from build123d import *

# Parameters (mm, degrees)
SKETCH1_R           = 2.6
BOSS_EXTRUDE1_DEPTH = 5
SKETCH2_W           = 69.749863317
SKETCH2_H           = 53.464567198
SKETCH2_W_2         = 56
SKETCH2_H_2         = 33
SKETCH2_R           = 13.5
CUT_EXTRUDE1_DEPTH  = 10
BOSS_EXTRUDE2_DEPTH = 5


with BuildPart() as part:
    # Sketch1 → Boss-Extrude1 (new body)
    with BuildSketch(Plane.XY):
        with BuildLine():
            Line((-28, -18.201493875), (-28, -24.201493875))
            Line((-28, -24.201493875), (28, -24.201493875))
            Line((28, -24.201493875), (28, -18.201493875))
            Line((28, -18.201493875), (26, -18.201493875))
            Line((26, -18.201493875), (26, -15.701493875))
            Line((26, -15.701493875), (23, -15.701493875))
            Line((23, -15.701493875), (23, -16.951493875))
            ThreePointArc((23, -16.951493875), (22, -17.951493875), (21, -16.951493875))
            Line((21, -16.951493875), (21, -15.701493875))
            Line((21, -15.701493875), (16, -15.701493875))
            Line((16, -15.701493875), (16, -12.701493875))
            Line((16, -12.701493875), (21, -12.701493875))
            Line((21, -12.701493875), (21, -11.451493875))
            ThreePointArc((21, -11.451493875), (22, -10.451493875), (23, -11.451493875))
            Line((23, -11.451493875), (23, -12.701493875))
            Line((23, -12.701493875), (26, -12.701493875))
            Line((26, -12.701493875), (26, -10.201493875))
            Line((26, -10.201493875), (28, -10.201493875))
            Line((28, -10.201493875), (28, -4.201493875))
            Line((28, -4.201493875), (26, -4.201493875))
            Line((26, -4.201493875), (26, 2.924352213))
            Line((26, 2.924352213), (12, 17.426918513))
            Line((12, 17.426918513), (-12, 17.426918513))
            Line((-12, 17.426918513), (-26, 2.924352213))
            Line((-26, 2.924352213), (-26, -4.201493875))
            Line((-26, -4.201493875), (-28, -4.201493875))
            Line((-28, -4.201493875), (-28, -10.201493875))
            Line((-28, -10.201493875), (-26, -10.201493875))
            Line((-26, -10.201493875), (-26, -12.701493875))
            Line((-26, -12.701493875), (-23, -12.701493875))
            Line((-23, -12.701493875), (-23, -11.451493875))
            ThreePointArc((-23, -11.451493875), (-22, -10.451493875), (-21, -11.451493875))
            Line((-21, -11.451493875), (-21, -12.701493875))
            Line((-21, -12.701493875), (-16, -12.701493875))
            Line((-16, -12.701493875), (-16, -15.701493875))
            Line((-16, -15.701493875), (-21, -15.701493875))
            Line((-21, -15.701493875), (-21, -16.951493875))
            ThreePointArc((-21, -16.951493875), (-22, -17.951493875), (-23, -16.951493875))
            Line((-23, -16.951493875), (-23, -15.701493875))
            Line((-23, -15.701493875), (-26, -15.701493875))
            Line((-26, -15.701493875), (-26, -18.201493875))
            Line((-26, -18.201493875), (-28, -18.201493875))
        make_face()
        with Locations((-21.5, -6.201493875)):
            Circle(SKETCH1_R, mode=Mode.SUBTRACT)
        with Locations((21.5, -6.201493875)):
            Circle(SKETCH1_R, mode=Mode.SUBTRACT)
        with BuildLine():
            Line((8.25, 3.201632482), (8.25, -1.451493875))
            Line((8.25, -1.451493875), (3.596873642, -1.451493875))
            ThreePointArc((3.596873642, -1.451493875), (0, -2.201493875), (-3.596873642, -1.451493875))
            Line((-3.596873642, -1.451493875), (-8.25, -1.451493875))
            Line((-8.25, -1.451493875), (-8.25, 3.201632482))
            ThreePointArc((-8.25, 3.201632482), (-8.626766656, 4.233570052), (-8.875, 5.303723532))
            ThreePointArc((-8.875, 5.303723532), (-10.25, 6.798506125), (-8.875, 8.293288717))
            ThreePointArc((-8.875, 8.293288717), (-8.626766656, 9.363442197), (-8.25, 10.395379767))
            Line((-8.25, 10.395379767), (-8.25, 15.048506125))
            Line((-8.25, 15.048506125), (-3.596873642, 15.048506125))
            ThreePointArc((-3.596873642, 15.048506125), (0, 15.798506125), (3.596873642, 15.048506125))
            Line((3.596873642, 15.048506125), (8.25, 15.048506125))
            Line((8.25, 15.048506125), (8.25, 10.395379767))
            ThreePointArc((8.25, 10.395379767), (8.626766656, 9.363442197), (8.875, 8.293288717))
            ThreePointArc((8.875, 8.293288717), (10.25, 6.798506125), (8.875, 5.303723532))
            ThreePointArc((8.875, 5.303723532), (8.626766656, 4.233570052), (8.25, 3.201632482))
        make_face(mode=Mode.SUBTRACT)
    extrude(amount=BOSS_EXTRUDE1_DEPTH)

    # Sketch2 → Cut-Extrude1 (cut)
    # profile 1 of 2: a face of its own
    with BuildSketch(Plane.XY.offset(5)):
        with Locations((5.197554668, -6.913421349)):
            Rectangle(SKETCH2_W, SKETCH2_H)
        with Locations((0, -14.201493875)):
            Rectangle(SKETCH2_W_2, SKETCH2_H_2, mode=Mode.SUBTRACT)
    # profile 2 of 2: a face of its own
    with BuildSketch(Plane.XY.offset(5)):
        with Locations((0, -14.201493875)):
            Circle(SKETCH2_R)
    extrude(amount=-CUT_EXTRUDE1_DEPTH, mode=Mode.SUBTRACT)


with BuildPart() as cut_extrude1_piece_1:
    # of the separate pieces the step leaves, piece 1, a body of its own (cut_extrude1_pieces)
    add(part.part.solids().sort_by_distance((9.069178574, -24.201493875, 0))[0])



with BuildPart() as cut_extrude1_piece_2:
    # of the separate pieces the step leaves, piece 2, a body of its own (cut_extrude1_pieces)
    add(part.part.solids().sort_by_distance((-28, -18.201493875, 0))[0])


with BuildPart() as cut_extrude1_piece_1_1:
    add(cut_extrude1_piece_1.part)

    add(cut_extrude1_piece_2.part)  # Boss-Extrude2 merges Cut-Extrude1 piece 2
    # Sketch3 → Boss-Extrude2 (add)
    with BuildSketch(Plane(origin=(0, 0, 0), x_dir=(-1, 0, 0), z_dir=(0, 0, -1))):
        with BuildLine():
            Line((-26, -4.201493875), (-26, -0.701493875))
            Line((-26, -0.701493875), (-26, 2.298506125))
            Line((-26, 2.298506125), (-8.25, 2.298506125))
            Line((-8.25, 2.298506125), (-8.25, -0.701493875))
            Line((-8.25, -0.701493875), (-8.25, -1.451493875))
            Line((-8.25, -1.451493875), (-4.437059837, -1.451493875))
            ThreePointArc((-4.437059837, -1.451493875), (2.167902598, -0.876697505), (8.25, -3.515638739))
            Line((8.25, -3.515638739), (8.25, -0.701493875))
            Line((8.25, -0.701493875), (26, -0.701493875))
            Line((26, -0.701493875), (26, -4.201493875))
            Line((26, -4.201493875), (28, -4.201493875))
            Line((28, -4.201493875), (28, -0.701493875))
            Line((28, -0.701493875), (28, 4.298506125))
            Line((28, 4.298506125), (-28.241259843, 4.298506125))
            Line((-28.241259843, 4.298506125), (-28.241259843, -0.701493875))
            Line((-28.241259843, -0.701493875), (-28.241259843, -4.201493875))
            Line((-28.241259843, -4.201493875), (-28, -4.201493875))
            Line((-28, -4.201493875), (-26, -4.201493875))
        make_face()
        Polygon((28, -27.701493875), (0, -27.701493875), (-28, -27.701493875), (-28, -32.701493875), (28, -32.701493875), align=None)
        with BuildLine():
            Line((28, -24.201493875), (9.069178574, -24.201493875))
            ThreePointArc((9.069178574, -24.201493875), (4.860555524, -26.796135593), (0, -27.701493875))
            Line((0, -27.701493875), (28, -27.701493875))
            Line((28, -27.701493875), (28, -24.201493875))
        make_face()
        with BuildLine():
            ThreePointArc((0, -27.701493875), (-4.860555524, -26.796135593), (-9.069178574, -24.201493875))
            Line((-9.069178574, -24.201493875), (-28, -24.201493875))
            Line((-28, -24.201493875), (-28, -27.701493875))
            Line((-28, -27.701493875), (0, -27.701493875))
        make_face()
    extrude(amount=-BOSS_EXTRUDE2_DEPTH)


solid = cut_extrude1_piece_1_1.part
Could you check a few things on this model? Use its own coordinates, in mm. A direction names the side the tool comes from. Coordinates: 2 decimals unless noted, no trailing zeros. Order: outer loops, then holes, each group sorted by start corner. A loop starts at its lowest first (then second) coordinate and runs counter-clockwise, first axis right, second up. Notation, with made-up numbers: (-28.5, 16.5) -> (4.5, 16.5) arc R37 ccw to (4.5, 54.5) -> close; hole circle Ø4 at (26, 75). An arc over 180 degrees is marked (long way). One line per question, with ' | ' between items.
Q1. Thinking about a two-plate mould opening in X: for faces 1 (the face through (21, -16, 2)), 2 (the face through (13, -10, 5)), 3 (the face through (16, -14, 2)), which applies, pulls with the +X half, pulls with the -X half, needs draft (parallel to the pull), parting line crosses it, or undercut?
Return value:
face 1: undercut | face 2: needs draft | face 3: pulls with the +X half
Q2. Imagine slicing it at C-C on y = -26. Please give me the cut outline in (x, z), and give its area (3 significant figures).
Return value:
outline: (-28, 0) -> (-6.56, 0) -> (-6.56, 5) -> (-28, 5) -> close; (6.56, 0) -> (28, 0) -> (28, 5) -> (6.56, 5) -> close | area: 214 mm²
Q3. Imagine slicing it at A-A on x = -11. Please give me the cut outline in (y, z), and give its area (3 significant figures).
Return value:
outline: (-32.7, 0) -> (-22.03, 0) -> (-22.03, 5) -> (-32.7, 5) -> close; (-6.38, 0) -> (4.3, 0) -> (4.3, 5) -> (-6.38, 5) -> close | area: 107 mm²
Q4. Imagine slicing it at D-D on z = 1.2. State how many separate pieces and enclosed holes the cut face has, and give its area (3 significant figures).
Return value:
separate pieces: 1 | enclosed holes: 3 | area: 1,350 mm²
Q5. I'm going to push flat-ended pins straight in: P1, Ø3, axis at y = -16.5, z = 1.5, coming from the +X side; P2, Ø1.5, axis at y = -14.5, z = 1.5, coming from the -X side; P3, Ø7, axis at x = 21.5, y = -6.2, coming from the -Z side; P4, Ø0.6, axis at y = -12.5, z = 1.5, coming from the -X side. Where does each tip first touch, or does it pass through?
Return value:
P1: x = 26 | P2: x = -16 | P3: z = 0 | P4: x = -26
Q6. If I drill on L1, parallel to Y at x = -21.5, z = 2; L2, parallel to Y at x = 20, z = 0.5; L3, parallel to X at y = -8.5, z = 4.7, over which ranges is the centre line in solid material (lowest first)?
Return value:
L1: -32.7 to -17.82, -10.59 to -8.8, -3.6 to 4.3 | L2: -32.7 to -15.7, -12.7 to -8.33, -4.08 to 4.3 | L3: -28 to -22.72, -20.28 to -12.24, 12.24 to 20.28, 22.72 to 28
Q7. On a 3-axis mill with a long thin cutter (end or side, diameter ignored), from which of +Z, -Z, +X, -X, +Y, -Y can I reach the whole of each face in a straight line? I mean faces 4 (the face through (-24, -15.701, 2)), 5 (the face through (26, -11, 2)), 6 (the face through (-23, -12, 2)). Say none if no direction works.
Return value:
face 4: +Z, -Z, -X | face 5: +Z, -Z, +X | face 6: +Z, -Z
Q8. Imagine slicing it at B-B on x = -19.5. Please give me the cut outline in (y, z).
Return value:
outline: (-32.7, 0) -> (-15.7, 0) -> (-15.7, 5) -> (-32.7, 5) -> close; (-12.7, 0) -> (-7.86, 0) -> (-7.86, 5) -> (-12.7, 5) -> close; (-4.54, 0) -> (4.3, 0) -> (4.3, 5) -> (-4.54, 5) -> close
